The model under review builds one solid part; all positions refer to its coordinate system, in mm. A direction names the side the tool comes from. Give positions to 0.01 mm unless a question says otherwise; leave off trailing zeros. Loops run counter-clockwise (first coordinate to the right, second up) from the corner with the lowest first, then second, coordinate; pieces in that order, holes last. Notation, with made-up numbers: M -20.5,22 L -16.5,22 A27 ccw -16.5,58 Z; hole C -35,15 d10. An arc over 180 degrees is marked long. Put each result on its own line as item: value. Start each with the question number.
Autodesk Inventor part; units mm, degrees
ref_plane "Arbeitsebene1" through (42.5, 0, 0) normal (1, 0, 0) x (0, 0, -1)
ref_plane "Arbeitsebene3" through (0, 0, 30) normal (0, 0, 1) x (1, 0, 0)
ref_plane "Arbeitsebene4" through (0, 0, 10) normal (0, 0, -1) x (-1, 0, 0)
sketch "Skizze1" plane through (0, 0, 0) normal (0, 0, 1) x (1, 0, 0)
  line L0 (0, 0) -> (50, 0)
  line L1 (50, 0) -> (50, 45)
  line L2 (35, 60) -> (15, 60)
  line L3 (0, 45) -> (0, 0)
  circle A0 centre (25, 28) radius 17.5
  line L4 (25, 28) -> (25, 0) construction
  line L5 (0, 45) -> (15, 60)
  line L6 (35, 60) -> (50, 45)
  line L7 (24, 60) -> (26, 60)
  line L8 (26, 60) -> (26, 28)
  line L9 (26, 28) -> (24, 28)
  line L10 (24, 28) -> (24, 60)
  point P0 (50, 60)
  point P1 (0, 60)
  point P2 (25, 60)
  dimension "d0" = 50
  dimension "d1" = 35
  dimension "d2" = 60
  dimension "d3" = 15
  dimension "d4" = 15
  dimension "d5" = 15
  dimension "d6" = 15
  dimension "d7" = 28
  dimension "d10" = 2
extrude "Extrusion1" add sketch "Skizze1" along normal blind 40 contours L3 L5 L2 L10 A0 L8 L6 L1 L0 | L2 L8 A0 L10
extrude "Extrusion2" cut sketch "Skizze1" along normal up to surface (40 mm away) contours L2 L8 A0 L10 | A0 L8 L9 L10 picked at (24.8888, 33.8323)
sketch "Skizze2" plane through (0, 0, 0) normal (0, -1, 0) x (1, 0, 0)
  line L0 (0, 0) -> (0, 40) construction
  line L1 (50, 0) -> (50, 40) construction
  line L2 (0, 40) -> (50, 40) construction
  line L3 (0, 0) -> (0, 40) construction
  line L4 (25, 20) -> (25, 40) construction
  line L5 (7.5, 40) -> (42.5, 40) construction
  line L6 (11, 20) -> (39, 20) construction
  point P0 (26, 40)
  point P1 (24, 40)
  point P2 (0, 20)
  dimension "d13" = 28
hole "Bohrung1" at (11, 0, 20) at (39, 0, 20) direction (0, 1, 0) diameter 2.459 depth 10 tip angle 118
ref_plane "Arbeitsebene1" through (42.5, 0, 0) normal (1, 0, 0) x (0, 0, -1)
sketch "Skizze3" plane through (42.5, 0, 0) normal (1, 0, 0) x (0, 0, -1)
  line L0 (0, 60) -> (-40, 60) construction
  line L1 (0, 45) -> (-40, 45) construction
  line L2 (-40, 45) -> (-40, 60) construction
  line L3 (-40, 52.5) -> (0, 52.5) construction
  line L4 (0, 45) -> (0, 60) construction
  point P0 (0, 0)
  point P1 (-20, 52.5)
  point P2 (-30, 52.5)
  point P3 (-10, 52.5)
  dimension "d44" = 10
  dimension "d45" = 10
ref_plane "Arbeitsebene2" through (0, 0, 20) normal (0, 0, 1) x (1, 0, 0)
ref_plane "Arbeitsebene3" through (0, 0, 30) normal (0, 0, 1) x (1, 0, 0)
ref_plane "Arbeitsebene4" through (0, 0, 10) normal (0, 0, -1) x (-1, 0, 0)
sketch "Skizze5" plane through (50, 0, 40) normal (1, 0, 0) x (0, 0, -1)
  line L0 (20, -12) -> (20, 72) construction
  line L1 (10, -12) -> (10, 72) construction
  line L2 (30, 72) -> (30, -12) construction
  point P0 (40, 0)
  dimension "Hole_Dist2Center" = 10
  dimension "d37" = 10
hole "Bohrung2" at (42.5, 52.5, 30) at (42.5, 52.5, 10) direction (-1, 0, 0) diameter 3.4 depth 18.5 counterbore diameter 6.5 counterbore depth 3.4
delete faces "Fläche löschen1" heal yes whole lump no faces at (42.5, 50.5955, 29.1479) (42.5, 51.6084, 10.6154)
sketch "Skizze4" plane through (24, 45.4714, 0) normal (1, 0, 0) x (0, 0, -1)
  line L0 (-20, 7.0286) -> (-30, 7.0286) construction
  line L1 (-30, -57.4714) -> (-30, 26.5286) construction
  line L2 (-10, 26.5286) -> (-10, -57.4714) construction
  point P0 (0, -45.4714)
  point P1 (-10, 7.0286)
hole "Bohrung3" at (24, 52.5, 30) at (24, 52.5, 10) direction (-1, 0, 0) diameter 3.242 end through all
equation "\"d0\" = Fixation_Width"
equation "\"d8\" = Fixation_Thickness"
equation "\"d11\" = Fixation_Thickness"
equation "\"d13\" = FixationHole_Dist"
equation "\"Fixation_Thickness\" = 40"
equation "\"Fixation_Width\" = 50"
equation "\"FixationHole_Dist\" = 28"
equation "\"d21\" = -0.5 * d5"
properties part number "Motor_ParallelMecha_Fixation_Holder"
Item 1: Draft analysis for pull direction X (two halves, no side actions). For faces 4 (the cylindrical face through (37.963, 5.07, 19.339)), 5 (the flat face through (31, 60, 20)), 6 (the flat face through (7, 52, 20)), state which applies: +X half, -X half, draft (parallel to the pull), parting line (faces both ways), or undercut.
Item 2: To check wall thickness, follow L1, parallel to Z at x = 35.25, y = 52.5; L2, parallel to X at y = 5.5, z = 20; L3, parallel to Z at x = 11.5, y = 52.5. State the ranges of each line that lie inside material, in increasing order. Write a range as [from, to].
Item 3: Tool access review of faces 1 (the flat face through (24, 53, 20)), 2 (the flat face through (42, 53, 20)), 3 (the cylindrical face through (41.644, 49.278, 30.423)): name each direction out of +Z, -Z, +X, -X, +Y, -Y from which nothing blocks a thin tool from reaching the whole face with its end or side.
Item 4: Consider section B-B, the plane y = 52.5. Give the number of separate pieces and of enclosed holes in the cut face, plus the area to 3 significant figures.
Item 5: Consider section C-C, the plane z = 30. Write out the cut boundary in (x, y), plus the area to 3 significant figures.
Item 6: Clearance check with flat-ended pins moving along their axes: pin 1 Ø1.5 at (x, z) = (11, 20) entering from +Y; pin 2 Ø6 at (y, z) = (52.5, 30) entering from +X; pin 3 Ø7 at (y, z) = (53.5, 9) entering from +X. State where each tip first meets the part, or that it passes through.
Item 7: Consider section A-A, the plane x = 33. Write out the cut boundary in (y, z), plus the area to 3 significant figures.
Item 8: Consider section D-D, the plane y = 43.5. Write out the cut boundary in (x, z), plus the area to 3 significant figures.
Report:
1. face 4: undercut
1. face 5: draft
1. face 6: -X half
2. L1: [0, 8.3], [11.7, 28.3], [31.7, 40]
2. L2: [0, 9.77], [12.23, 37.77], [40.23, 50]
2. L3: [0, 8.38], [11.62, 28.38], [31.62, 40]
3. face 1: +Z, -Z, +Y
3. face 2: +Z, -Z, +X, +Y
3. face 3: +X
4. separate pieces: 6
4. enclosed holes: 0
4. area: 1,080 mm²
5. outline: M 0,0 L 50,0 L 50,45 L 45.75,49.25 L 39.1,49.25 L 39.1,50.8 L 26,50.8 L 26,45.47 A17.5 cw long 24,45.47 L 24,50.88 L 5.88,50.88 L 0,45 Z; M 9.12,54.12 L 24,54.12 L 24,60 L 15,60 Z; M 26,54.2 L 39.1,54.2 L 39.1,55.75 L 39.25,55.75 L 35,60 L 26,60 Z
5. area: 1,660 mm²
6. pin 1: y = 56.75
6. pin 2: x = 39.1
6. pin 3: x = 44.72
7. outline: M 0,0 L 12.44,0 L 12.44,40 L 0,40 Z; M 43.56,0 L 60,0 L 60,40 L 43.56,40 Z; hole C 52.5,10 d3.4; hole C 52.5,30 d3.4
7. area: 1,140 mm²
8. outline: M 0,0 L 16.88,0 L 16.88,40 L 0,40 Z; M 33.12,0 L 50,0 L 50,40 L 33.12,40 Z
8. area: 1,350 mm²
